Input: part model. Units: mm. Frame: model coordinates. Coordinates: 2 decimals unless noted, no trailing zeros. Loops run counter-clockwise (first coordinate to the right, second up) from the corner with the lowest first, then second, coordinate; pieces in that order, holes last. Notation, with made-up numbers: M -20,79.25 L -1,79.25 A15 ccw -1,106.25 Z; hole C 17,-27 d8. An arc over 180 degrees is marked long. Use a Markdown table: item, result. Add a question column.
1. Pin query (flat end, axial travel): pin 1 (1.5 mm diameter, centred on x = -1, y = 9, fed in from +Z). Return the tip coordinate at first contact, or that it passes through.
2. Section C-C on z = 154. Output: boundary loops of the cut face in (x, y).
3. Section A-A on x = -1.95. Output: boundary loops of the cut face in (y, z).
4. Line query: L1, parallel to Y at x = -0.6, z = 131; L2, parallel to Y at x = -2.85, z = 614.5; L3, parallel to Z at x = -2.05, y = 6. Output: solid intervals per line, ascending. Write a range as [from, to].
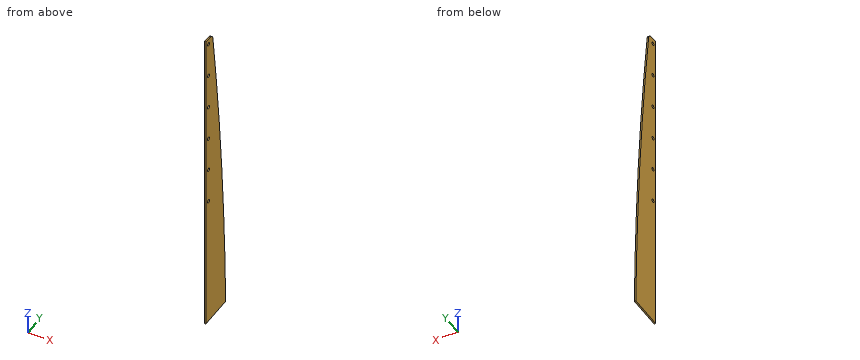
Autodesk Inventor part; units mm, degrees
ref_plane "YZ Plane" through (0, 0, 0) normal (1, 0, 0) x (0, 1, 0)
ref_plane "XZ Plane" through (0, 0, 0) normal (0, 1, 0) x (-1, 0, 0)
ref_plane "XY Plane" through (0, 0, 0) normal (0, 0, 1) x (1, 0, 0)
sketch "Sketch1" plane through (0, 0, 0) normal (1, 0, 0) x (0, 1, 0)
  line L0 (25, 748.8121) -> (0, 748.8121)
  line L1 (0, 748.8121) -> (0, -748.8121)
  line L2 (0, -748.8121) -> (25, -748.8121)
  arc A0 (25, -748.8121) -> (25, 748.8121) centre (-5575.159, 0) ccw
  line L3 (0, 748.8121) -> (25.2835, 746.689)
  line L4 (0, -748.8121) -> (25.2835, -746.689)
  line L5 (0, 97) -> (74.0083, 97)
  point P0 (0, 0)
  point P1 (0, 0)
  dimension "d2" = 25
  dimension "d3" = 5650
  dimension "d7" = 85.2
  dimension "d8" = 85.2
  dimension "d33" = 97
  dimension "d34" = 651.812
extrude "Plate1" add sketch "Sketch1" against normal blind 3.048 contours L3 A0 L5 L1
fillet "Corner Round3" radius 10 1 edges at (-1.524, 25.2835, 746.689)
sketch "Sketch4" plane through (0, 0, 0) normal (1, 0, 0) x (0, 0, -1)
  circle A0 centre (-735.8121, 10) radius 3.5
  line L0 (-748.8121, 0) -> (-97, 0)
  point P0 (0, 0)
  dimension "d23" = 7
  dimension "d25" = 10
  dimension "d32" = 13
extrude "Extrusion1" cut sketch "Sketch4" against normal through all
pattern_linear "Rectangular Pattern2" count 6 spacing 72.5 along (0, 0, -1) of "Extrusion1"
equation "\"BendReliefWidth\" = Thickness"
equation "\"BendReliefDepth\" = 0.5 * Thickness"
equation "\"CornerReliefSize\" = 4 * Thickness"
equation "\"MinimumRemnant\" = 2 * Thickness"
equation "\"TransitionRadius\" = BendRadius"
equation "\"JacobiRadiusSize\" = BendRadius"
equation "\"GapSize\" = Thickness"
equation "\"BendRadius\" = Thickness"
properties part number "MSC 083 top support gills" material "Stainless Steel"
Answers below:
| question | item | result |
|---|---|---|
| 1 | pin 1 | stops at z = 748.12 |
| 2 | outline | M -3.05,0 L 0,0 L 0,72.74 L -3.05,72.74 Z |
| 3 | outline | M 0,97 L 74.01,97 A5650 ccw 26.34,738.7 A10 ccw 17.26,747.36 L 0,748.81 Z; hole C 10,373.31 d7; hole C 10,445.81 d7; hole C 10,518.31 d7; hole C 10,590.81 d7; hole C 10,663.31 d7; hole C 10,735.81 d7 |
| 4 | L1 | y = [0, 73.32] |
| 4 | L2 | y = [0, 41.32] |
| 4 | L3 | z = [97, 748.31] |
